For this review, take the finished solid that the model builds, in its own axes (mm). Face numbers are marked on the shaded views. A direction names the side the tool comes from. Round coordinates to 2 decimals unless told otherwise and drop trailing zeros. Write each loop counter-clockwise with the first axis right and the second up, starting at its lowest first coordinate (ties: lowest second). Pieces come first, ordered by that corner, then holes. Notation, with made-up numbers: (19.25, 14.5) - (60.25, 14.5) arc R19 cw to (60.25, 49.5) - close; hole circle Ø3 at (58.25, 11). An arc over 180 degrees is marked (long way). One line per item, written item: value. Start each with the question number.
Q1. Add section A-A on z = 4. Write out the cut boundary in (x, y), and give its area (3 significant figures).
Q2. Tool access review of the marked faces 1 and 2: name each direction out of +Z, -Z, +X, -X, +Y, -Y from which nothing blocks a thin tool from reaching the whole face with its end or side.
Q3. For probe 1 along Z at (x, y) = (47.5, 24.75); probe 2 along X at (y, z) = (22.75, 8.5); probe 3 along Z at (x, y) = (26.05, 13), list the stretches that pass through material, from the lowest coordinate up.
Q4. Add section B-B on z = 12.25. Write out the cut boundary in (x, y).
Q5. Clearance check with flat-ended pins moving along their axes: pin 1 Ø5 at (x, z) = (46.5, 7.5) entering from -Y; pin 2 Ø1.5 at (x, z) = (27, 4.5) entering from +Y; pin 3 Ø3.5 at (x, z) = (65, 1) entering from -Y; pin 4 Ø5 at (y, z) = (13, 8) entering from +X. State where each tip first meets the part, or that it passes through.
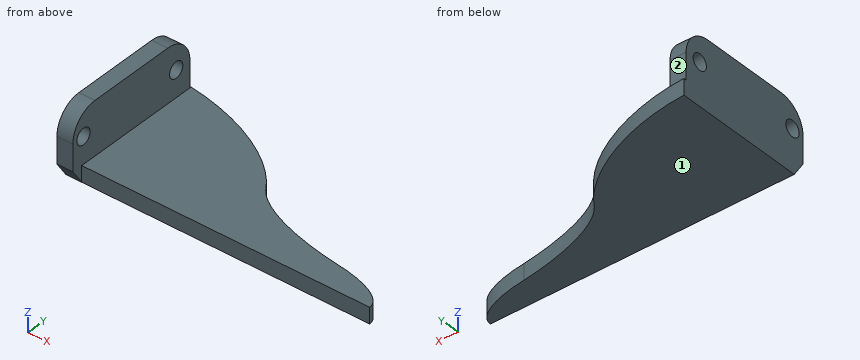
```python
from build123d import *

# Parameters (mm, degrees)
PAD_DEPTH    = 3
SKETCH001_W  = 26.5
SKETCH001_H  = 10
PAD001_DEPTH = 3
SKETCH002_R  = 1.5
POCKET_DEPTH = 57.001
PAD002_DEPTH = 3
FILLET_R     = 5


with BuildPart() as part:
    # Sketch → Pad (new body)
    with BuildSketch(Plane.XY):
        with BuildLine():
            add(Edge.make_bspline(
                [(51.853295, 25.571163), (55.204896, 19.874189), (71.483399, 17.693641)],
                knots=[0.193341, 0.193341, 0.193341, 1.192921, 1.192921, 1.192921], degree=2, weights=[1, 0.877683, 1]))
            add(Edge.make_bspline(
                [(82, 12.6), (82, 16.588456), (71.483399, 17.693641)],
                knots=[0, 0, 0, 1.290026, 1.290026, 1.290026], degree=2, weights=[1, 0.799092, 1]))
            Line((82, 12.6), (25, 12.6))
            Line((25, 12.6), (25, 37.6))
            add(Edge.make_bspline(
                [(51.853295, 25.571163), (43.781474, 36.750026), (25, 37.6)],
                knots=[0.559519, 0.559519, 0.559519, 1.875492, 1.875492, 1.875492], degree=2, weights=[1, 0.791225, 1]))
        make_face()
    extrude(amount=PAD_DEPTH)

    # Sketch001 (on Face4 of Pad) → Pad001 (join)
    with BuildSketch(Plane(origin=(25, 0, 0), x_dir=(0, -1, 0), z_dir=(-1, 0, 0))):
        with Locations((-23.85, 8)):
            Rectangle(SKETCH001_W, SKETCH001_H)
    extrude(amount=-PAD001_DEPTH)

    # Sketch002 (on Face10 of Pad001) → Pocket (cut, through all)
    with BuildSketch(Plane(origin=(25, 0, 0), x_dir=(0, -1, 0), z_dir=(-1, 0, 0))):
        with Locations((-34, 8)):
            Circle(SKETCH002_R)
        with Locations((-13, 8)):
            Circle(SKETCH002_R)
    extrude(amount=-POCKET_DEPTH, mode=Mode.SUBTRACT)

    # Sketch003 (on Face6 of Pocket) → Pad002 (join)
    with BuildSketch(Plane(origin=(25, 0, 0), x_dir=(0, -1, 0), z_dir=(-1, 0, 0))):
        Polygon((-12.6, 0), (-10.6, 3), (-12.6, 3), align=None)
    extrude(amount=-PAD002_DEPTH)

    # Fillet
    fillet_edges = [part.edges().sort_by_distance(p)[0] for p in [
        (26.5, 10.6, 13),
        (26.5, 37.1, 13),
    ]]
    fillet(fillet_edges, radius=FILLET_R)


solid = part.part
```
Result set:
1. outline: (25, 10.6) - (28, 10.6) - (28, 37.1) - (25, 37.1) - close
1. area: 79.5 mm^2
2. face 1: -Z, +X, -X, +Y, -Y
2. face 2: +Z, +X, -X, +Y
3. probe 1: z = 0 to 3
3. probe 2: x = 25 to 28
3. probe 3: z = 0 to 6.5, 9.5 to 12.27
4. outline: (25, 12.97) - (28, 12.97) - (28, 34.73) - (25, 34.73) - close
5. pin 1: passes through
5. pin 2: stops at y = 37.1
5. pin 3: stops at y = 12.6
5. pin 4: stops at x = 28
